Geometry check sheet. Reference: the model listing, model coordinates, mm. Face numbers are marked on the shaded views. A direction names the side the tool comes from. Give positions to 0.01 mm unless a question says otherwise; leave off trailing zeros. Loops run counter-clockwise (first coordinate to the right, second up) from the corner with the lowest first, then second, coordinate; pieces in that order, holes last. Notation, with made-up numbers: (16, 67.5) - (64, 67.5) arc R20 ccw to (64, 83.5) - close; hole circle Ø8 at (-8, 20.5). An arc over 180 degrees is marked (long way). Use a Markdown table: item, result. Add a question column.
1. Cross-section at A-A on z = 0. Enter the section's corners in (x, y).
2. Cross-section at C-C on x = 0. Enter the section's corners in (y, z).
3. Set-up check for the marked faces 4 and 5: record each of +Z, -Z, +X, -X, +Y, -Y from which the full face is reachable in a straight line by a thin tool's end or side.
4. Cross-section at D-D on z = 20.5. Enter the section's corners in (x, y).
5. Draft check along X on the marked faces 1, 2 and 3. Enter one of: pulls with the +X half, pulls with the -X half, needs draft (parallel to the pull), parting line crosses it, or undercut.
6. Material ranges on L1, parallel to X at y = -3.5, z = 0; L2, parallel to Z at x = 13, y = 2.5; L3, parallel to Z at x = -12, y = -6, recorded low to high.
7. Depth check by flat-ended pin: P1, Ø2, axis at y = 3, z = 0, coming from the +X side; P2, Ø1.7, axis at x = -11.5, z = -17, coming from the +Y side; P3, Ø3, axis at x = 11, z = 17.5, coming from the +Y side; P4, Ø12, axis at y = -2.5, z = 21, coming from the +X side. Enter the tip coordinate at first touch or a pass-through.
8. Cross-section at B-B on y = 6.5. Enter the section's corners in (x, z).
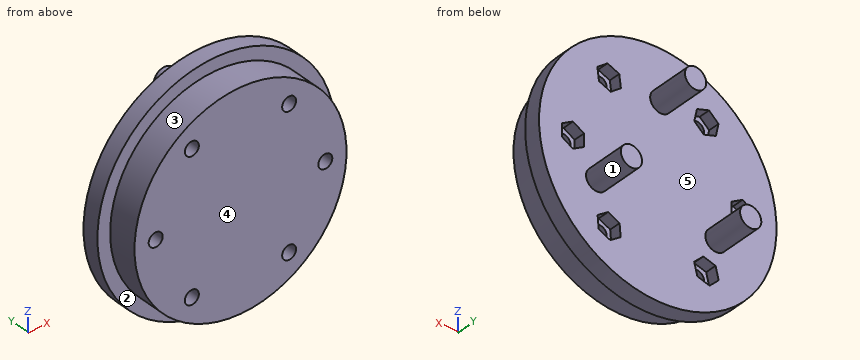
from build123d import *

# Parameters (mm, degrees)
SKETCH3_R               = 28
BOSS_EXTRUDE1_DEPTH     = 4
SKETCH6_R               = 25
BOSS_EXTRUDE4_DEPTH     = 7
SKETCH7_R               = 2.5
BOSS_EXTRUDE5_DEPTH     = 10
CUT_EXTRUDE1_DEPTH      = 10
CUT_EXTRUDE1_DEPTH_BACK = 43
SKETCH8_R               = 1.65
CUT_EXTRUDE3_DEPTH      = 2.7


with BuildPart() as part:
    # Sketch3 → Boss-Extrude1 (new body)
    with BuildSketch(Plane(origin=(0, 0, 0), x_dir=(1, 0, 0), z_dir=(0, 1, 0))):
        with Locations(Location((0, 0, 0), (0, 0, 270))):
            Circle(SKETCH3_R)
    extrude(amount=BOSS_EXTRUDE1_DEPTH)

    # Sketch6 → Boss-Extrude4 (add)
    with BuildSketch(Plane.XZ):
        with Locations(Location((0, 0, 0), (0, 0, 270))):
            Circle(SKETCH6_R)
    extrude(amount=BOSS_EXTRUDE4_DEPTH)

    # Sketch7 → Boss-Extrude5 (add)
    with BuildSketch(Plane(origin=(0, 4, 0), x_dir=(1, 0, 0), z_dir=(0, 1, 0))):
        with Locations(Location((14.413926039, 7.503414965, 0), (0, 0, 270))):
            Circle(SKETCH7_R)
        with Locations(Location((-13.705110994, 8.731118636, 0), (0, 0, 270))):
            Circle(SKETCH7_R)
        with Locations(Location((-0.708815045, -16.234533601, 0), (0, 0, 270))):
            Circle(SKETCH7_R)
    extrude(amount=BOSS_EXTRUDE5_DEPTH)

    # Sketch8 → Cut-Extrude1 (cut, two sides: drawn at the far end of the back side and taken through both)
    with BuildSketch(Plane.XZ.offset(-CUT_EXTRUDE1_DEPTH_BACK)):
        with Locations(Location((20, 0, 0), (0, 0, 90))):
            Circle(SKETCH8_R)
        with Locations(Location((-20, 0, 0), (0, 0, 90))):
            Circle(SKETCH8_R)
        with Locations(Location((11.471528727, 16.383040886, 0), (0, 0, 90))):
            Circle(SKETCH8_R)
        with Locations(Location((-11.471528727, -16.383040886, 0), (0, 0, 90))):
            Circle(SKETCH8_R)
        with Locations(Location((11.471528727, -16.383040886, 0), (0, 0, 90))):
            Circle(SKETCH8_R)
        with Locations(Location((-11.471528727, 16.383040886, 0), (0, 0, 90))):
            Circle(SKETCH8_R)
    extrude(amount=CUT_EXTRUDE1_DEPTH + CUT_EXTRUDE1_DEPTH_BACK, mode=Mode.SUBTRACT)

    # Sketch11 → Cut-Extrude3 (cut)
    with BuildSketch(Plane(origin=(0, 4, 0), x_dir=(1, 0, 0), z_dir=(0, 1, 0))):
        Polygon((11.858091258, -19.360271603), (14.243167426, -17.536883273), (13.856604896, -14.559652555), (11.084966196, -13.405810169), (8.699890028, -15.229198499), (9.086452558, -18.206429216), align=None)
        Polygon((-12.091418901, -19.320568674), (-9.237500125, -18.388645418), (-8.617609951, -15.45111763), (-10.851638553, -13.445513098), (-13.705557329, -14.377436353), (-14.325447503, -17.314964141), align=None)
        Polygon((-22.590586111, -1.517299224), (-19.981273382, -3.002162995), (-17.390687271, -1.48486377), (-17.409413889, 1.517299224), (-20.018726618, 3.002162995), (-22.609312729, 1.48486377), align=None)
        Polygon((20, -3.0022214), (22.6, -1.5011107), (22.6, 1.5011107), (20, 3.0022214), (17.4, 1.5011107), (17.4, -1.5011107), align=None)
        Polygon((9.008253879, 14.666762832), (11.726231698, 13.391643264), (14.189506546, 15.107921318), (13.934803575, 18.09931894), (11.216825756, 19.374438507), (8.753550908, 17.658160453), align=None)
        Polygon((-10.729703857, 13.473912288), (-8.581237024, 15.57091577), (-9.323061894, 18.480044367), (-12.213353597, 19.292169483), (-14.36182043, 17.195166002), (-13.61999556, 14.286037405), align=None)
    extrude(amount=-CUT_EXTRUDE3_DEPTH, mode=Mode.SUBTRACT)


solid = part.part
Values found:
| question | item | result |
|---|---|---|
| 1 | outline | (-28, 0) - (-25, 0) - (-25, -7) - (-21.65, -7) - (-21.65, 1.3) - (-22.6, 1.3) - (-22.6, 4) - (-28, 4) - close; (-18.35, -7) - (18.35, -7) - (18.35, 1.3) - (17.4, 1.3) - (17.4, 4) - (-17.4, 4) - (-17.4, 1.3) - (-18.35, 1.3) - close; (21.65, -7) - (25, -7) - (25, 0) - (28, 0) - (28, 4) - (22.6, 4) - (22.6, 1.3) - (21.65, 1.3) - close |
| 2 | outline | (-7, -25) - (0, -25) - (0, -28) - (4, -28) - (4, 13.84) - (14, 13.84) - (14, 18.63) - (4, 18.63) - (4, 28) - (0, 28) - (0, 25) - (-7, 25) - close |
| 3 | face 4 | +Z, -Z, +X, -X, -Y |
| 3 | face 5 | +Y |
| 4 | outline | (-19.07, 0) - (-14.31, 0) - (-14.31, -7) - (14.31, -7) - (14.31, 0) - (19.07, 0) - (19.07, 4) - (-19.07, 4) - close |
| 5 | face 1 | undercut |
| 5 | face 2 | needs draft |
| 5 | face 3 | parting line crosses it |
| 6 | L1 | x = -25 to -21.65, -18.35 to 18.35, 21.65 to 25 |
| 6 | L2 | z = -24.8 to -18.54, -14.28 to 14.2, 18.49 to 24.8 |
| 6 | L3 | z = -21.93 to -17.95, -14.82 to 14.82, 17.95 to 21.93 |
| 7 | P1 | stops at x = 28 |
| 7 | P2 | passes through |
| 7 | P3 | stops at y = 4 |
| 7 | P4 | stops at x = 23.29 |
| 8 | outline | circle Ø5 at (-13.71, -8.73); circle Ø5 at (-0.71, 16.23); circle Ø5 at (14.41, -7.5) |
